from build123d import *

# Parameters (mm, degrees)
SKETCH_1_R          = 2.5
EXTRUDE_1_DEPTH     = 8
SKETCH_2_R          = 1.5
CUT_EXTRUDE_1_DEPTH = 10
FILLET_1_R          = 3


with BuildPart() as part:
    # 草图1 → 凸台-拉伸1 (new body)
    with BuildSketch(Plane.XY):
        with BuildLine():
            Line((-10, 0), (10, 0))
            Line((10, 0), (10, 6))
            Line((10, 6), (7.957956343, 21.647046293))
            ThreePointArc((7.957956343, 21.647046293), (3.820468041, 25.932223859), (-1.481479577, 23.2172823))
            Line((-1.481479577, 23.2172823), (-10, 6))
            Line((-10, 6), (-10, 0))
        make_face()
        with Locations((3, 21)):
            Circle(SKETCH_1_R, mode=Mode.SUBTRACT)
    extrude(amount=EXTRUDE_1_DEPTH)

    # 草图2 → 切除-拉伸1 (cut)
    with BuildSketch(Plane.XZ):
        with Locations((-6, 4)):
            Circle(SKETCH_2_R)
        with Locations((6, 4)):
            Circle(SKETCH_2_R)
    extrude(amount=-CUT_EXTRUDE_1_DEPTH, mode=Mode.SUBTRACT)

    # 圆角1
    fillet_1_edges = [part.edges().sort_by_distance(p)[0] for p in [
        (-10, 6, 4),
        (10, 6, 4),
    ]]
    fillet(fillet_1_edges, radius=FILLET_1_R)


solid = part.part
For this review, take the finished solid that the model builds, in its own axes (mm). A direction names the side the tool comes from. Round coordinates to 2 decimals unless told otherwise and drop trailing zeros. Order: outer loops, then holes, each group sorted by start corner. A loop starts at its lowest first (then second) coordinate and runs counter-clockwise, first axis right, second up. Notation, with made-up numbers: M 85,-3.5 L 121,-3.5 A17 cw 121,26.5 Z; hole C 63,-38 d9. An arc over 180 degrees is marked long. Use a Markdown table: item, result. Add a question column.
Item 1: Tool access review of faces 1 (the flat face through (6, 10, 4)), 2 (the cylindrical face through (-9.923, 5.972, 4.056)): name each direction out of +Z, -Z, +X, -X, +Y, -Y from which nothing blocks a thin tool from reaching the whole face with its end or side.
Item 2: Add section C-C, the plane x = 6. Give the boundary of the cut face in (y, z), then the cut area to 3 significant figures.
Item 3: Insertion check: pin 1 (3 mm diameter, centred on x = 0.5, z = 5.5, fed in from +Y); pin 2 (4 mm diameter, centred on x = -6, z = 4, fed in from -Y); pin 3 (2.5 mm diameter, centred on x = 6, z = 4, fed in from +Y); pin 4 (3 mm diameter, centred on x = -2.5, z = 6.5, fed in from +Y). Each pin has a flat end and moves straight along its axis. Give the tip position at first contact, or say it passes through.
Item 4: To check wall thickness, follow line 1 along Y through (x, z) = (3, 5); line 2 along Z through (x, y) = (6, 3.5); line 3 along X through (y, z) = (3.5, 2.75). State the ranges of each line that lie inside material, in increasing order.
Item 5: Add section B-B, the plane z = 4. Give the boundary of the cut face in (x, y).
Item 6: Add section A-A, the plane y = 21. Give the boundary of the cut face in (x, z).
Item 7: Mouldability with a two-part tool opening along Y and no side actions: class faces 3 (the flat face through (-5.528, 15.039, 3.944)), 4 (the flat face through (0, 0, 4)), 5 (the cylindrical face through (2.67, 23.48, 3.94)) as released by +Y, released by -Y, zero draft, split by the parting line, or undercut.
Item 8: Add section D-D, the plane y = 8. Give the boundary of the cut face in (x, z), then the cut area to 3 significant figures.
Geometry results:
| question | item | result |
|---|---|---|
| 1 | face 1 | -Y |
| 1 | face 2 | +Z, -Z, -X, +Y |
| 2 | outline | M 0,0 L 25,0 L 25,8 L 0,8 L 0,5.5 L 10,5.5 L 10,2.5 L 0,2.5 Z |
| 2 | area | 170 mm² |
| 3 | pin 1 | stops at y = 25.9 |
| 3 | pin 2 | stops at y = 0 |
| 3 | pin 3 | stops at y = 25.68 |
| 3 | pin 4 | stops at y = 24 |
| 4 | line 1 | y = 0 to 18.5, 23.5 to 26 |
| 4 | line 2 | z = 0 to 2.5, 5.5 to 8 |
| 4 | line 3 | x = -10 to -6.83, -5.17 to 5.17, 6.83 to 10 |
| 5 | outline | M -10,0 L -7.5,0 L -7.5,10 L -4.5,10 L -4.5,0 L 4.5,0 L 4.5,10 L 7.5,10 L 7.5,0 L 10,0 L 10,5.81 A3 ccw 9.97,6.19 L 7.96,21.65 A5 ccw -1.48,23.22 L -9.69,6.63 A3 ccw -10,5.3 Z; hole C 3,21 d5 |
| 6 | outline | M -2.58,0 L 0.5,0 L 0.5,8 L -2.58,8 Z; M 5.5,0 L 8.04,0 L 8.04,8 L 5.5,8 Z |
| 7 | face 3 | released by +Y |
| 7 | face 4 | released by -Y |
| 7 | face 5 | undercut |
| 8 | outline | M -9.01,0 L 9.74,0 L 9.74,8 L -9.01,8 Z; hole C -6,4 d3; hole C 6,4 d3 |
| 8 | area | 136 mm² |
